Input: dimensioned drawing with shaded views. Units: mm. Origin: part minimum x, y, z. A direction names the side the tool comes from. Give positions to 0.01 mm unless a question says otherwise; leave off trailing zeros. Write each loop counter-clockwise with the first axis right and the second up, starting at its lowest first coordinate (ties: lowest second). Pieces come first, ordered by that corner, then holes. Notation, with made-up numbers: M 70,-25.5 L 96,-25.5 A22 ccw 96,-6.5 Z; hole C 67.5,33.25 d7. An arc over 180 degrees is marked long. Use CSV: the item, a comma, the result in double quotes. Start each with the question number.
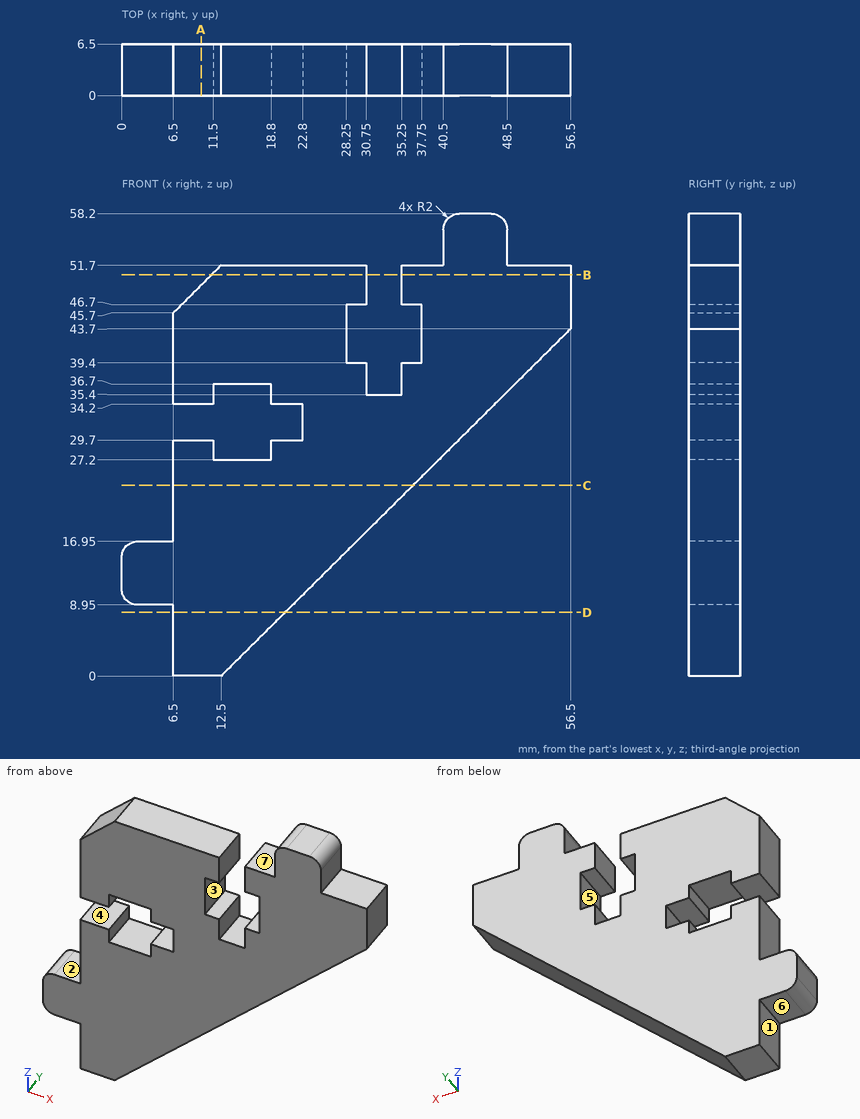
Q1. Section B-B, the plane z = 50.5. Return the cut outline in (x, y), and give its area (3 significant figures).
Q2. Set-up query: the marked faces 1, 2, 3 and 4. Return all of +Z, -Z, +X, -X, +Y, -Y with unobstructed straight access to the full face (end or side cutting, diameter ignored); none if empty.
Q3. First-contact query: pin 1 Ø1.6 at (x, y) = (38.5, 4) entering from +Z; pin 2 Ø1 at (x, y) = (46.5, 2.5) entering from -Z; pin 3 Ø2.5 at (y, z) = (4.5, 48) entering from -X. Flat tips, straight axial feed; report the tip coordinate or a pass-through.
Q4. Material intervals for L1, parallel to X at y = 6, z = 44.5; L2, parallel to X at y = 5.75, z = 36.5; L3, parallel to Z at x = 5.5, y = 2.75, sorted ascending. Write a range as [from, to].
Q5. Section A-A, the plane x = 10. Return the cut outline in (y, z), and give its area (3 significant figures).
Q6. Pull-direction query (Z, two-part tool) for the marked faces 5, 6 and 7; classes: released by +Z, released by -Z, zero draft, split by the parting line, or undercut.
Q7. Section C-C, the plane z = 24. Return the cut outline in (x, y), and give its area (3 significant figures).
Q8. Section D-D, the plane z = 8. Return the cut outline in (x, y), and give its area (3 significant figures).
Check result:
1,outline,"M 11.3,0 L 30.75,0 L 30.75,6.5 L 11.3,6.5 Z; M 35.25,0 L 56.5,0 L 56.5,6.5 L 35.25,6.5 Z"
1,area,"265 mm²"
2,face 1,"-Z, -X, +Y, -Y"
2,face 2,"+Z, -X, +Y, -Y"
2,face 3,"+Y, -Y"
2,face 4,"-X, +Y, -Y"
3,pin 1,"stops at z = 51.7"
3,pin 2,"stops at z = 33.27"
3,pin 3,"stops at x = 7.55"
4,L1,"x = [6.5, 28.25], [37.75, 56.5]"
4,L2,"x = [6.5, 11.5], [18.8, 30.75], [35.25, 49.25]"
4,L3,"z = [8.95, 16.95]"
5,outline,"M 0,0 L 6.5,0 L 6.5,29.7 L 0,29.7 Z; M 0,34.2 L 6.5,34.2 L 6.5,49.2 L 0,49.2 Z"
5,area,"291 mm²"
6,face 5,"undercut"
6,face 6,"released by -Z"
6,face 7,"released by +Z"
7,outline,"M 6.5,0 L 36.66,0 L 36.66,6.5 L 6.5,6.5 Z"
7,area,"196 mm²"
8,outline,"M 6.5,0 L 20.55,0 L 20.55,6.5 L 6.5,6.5 Z"
8,area,"91.4 mm²"
